Input: part model. Units: mm. Frame: model coordinates. A direction names the side the tool comes from. Give positions to 0.01 mm unless a question says otherwise; leave off trailing zeros. Order: outer loops, then holes, each group sorted by start corner. A loop starts at its lowest first (then second) coordinate and runs counter-clockwise, first axis right, second up. Notation, with made-up numbers: (-4, 64.25) - (20, 64.25) arc R26 ccw to (20, 95.25) - close; hole circle Ø4 at (3.5, 37.25). An arc over 180 degrees is marked (long way). Answer in a Markdown table with one row per item. Add a question column.
from build123d import *

# Parameters (mm, degrees)
CHAMFER_1_SIZE = 1.5


with BuildPart() as part:
    # Эскиз1 → Повернуть1 (revolve)
    with BuildSketch(Plane(origin=(0, 0, 0), x_dir=(0, 0, -1), z_dir=(1, 0, 0))):
        Polygon((-15, 0), (-28.5, 0), (-28.5, 19), (-23.5, 19), (-23.5, 5), (-11, 5), (-11, -5), (-15, -5), align=None)
    revolve(axis=Axis((0, 19.771159875, 0), (0, -1, 0)))

    # Фаска1
    chamfer_1_edges = [part.edges().sort_by_distance(p)[0] for p in [
        (0, 19, -28.5),
        (0, 0, -28.5),
        (0, -5, -15),
    ]]
    chamfer(chamfer_1_edges, length=CHAMFER_1_SIZE)


solid = part.part
Q1. Section C-C, the plane y = 15. Return loops of the section in (x, z).
Q2. Pull-direction query (Z, two-part tool) for faces 3 (the cylindrical face through (-0.66, -1.726, -14.985)), 4 (the flat face through (12, 0, -12)), 5 (the cylindrical face through (10.74, -0.07, -2.38)), 6 (the flat face through (5, 5, 10)); classes: +Z half, -Z half, draft (parallel to the pull), parting line (faces both ways), or undercut.
Q3. Section A-A, the plane x = 0. Return loops of the section in (y, z).
Q4. Access query for faces 1 (the cylindrical face through (-7.1, 11.9, 22.4)), 2 (the cylindrical face through (10.916, 9.612, 26.327)). Directions: +Z, -Z, +X, -X, +Y, -Y. A direction counts if a zero-diameter tool reaches every point of the face in a straight line with its end or side. Return the directions, or none.
Q5. Line query: probe 1 along Z at (x, y) = (0, 12); probe 2 along Z at (x, y) = (0, -1). Output: solid intervals per line, ascending.
Q6. Contact query for flat-ended pins moving along their axis: P1, Ø4, axis at x = 20, z = 14, coming from the -Y side; P2, Ø10, axis at y = 15, z = 18.5, coming from the +X side; P3, Ø6, axis at y = -1, z = -7, coming from the +X side; P4, Ø20, axis at x = 0, z = 0, coming from the +Y side. Output: stop coordinate, or through.
Q7. Section B-B, the plane z = 0. Return loops of the section in (x, y), then the cut area to 3 significant figures.
Computed:
| question | item | result |
|---|---|---|
| 1 | outline | circle Ø57 at (0, 0); hole circle Ø47 at (0, 0) |
| 2 | face 3 | parting line |
| 2 | face 4 | draft |
| 2 | face 5 | undercut |
| 2 | face 6 | undercut |
| 3 | outline | (-5, -13.5) - (-3.5, -15) - (0, -15) - (0, -27) - (1.5, -28.5) - (17.5, -28.5) - (19, -27) - (19, -23.5) - (5, -23.5) - (5, -11) - (-5, -11) - close; (-5, 11) - (5, 11) - (5, 23.5) - (19, 23.5) - (19, 27) - (17.5, 28.5) - (1.5, 28.5) - (0, 27) - (0, 15) - (-3.5, 15) - (-5, 13.5) - close |
| 4 | face 1 | +Y |
| 4 | face 2 | +Y, -Y |
| 5 | probe 1 | z = -28.5 to -23.5, 23.5 to 28.5 |
| 5 | probe 2 | z = -15 to -11, 11 to 15 |
| 6 | P1 | stops at y = 0 |
| 6 | P2 | stops at x = 25.1 |
| 6 | P3 | stops at x = 27.99 |
| 6 | P4 | passes through |
| 7 | outline | (-28.5, 1.5) - (-27, 0) - (-15, 0) - (-15, -3.5) - (-13.5, -5) - (-11, -5) - (-11, 5) - (-23.5, 5) - (-23.5, 19) - (-27, 19) - (-28.5, 17.5) - close; (11, -5) - (13.5, -5) - (15, -3.5) - (15, 0) - (27, 0) - (28.5, 1.5) - (28.5, 17.5) - (27, 19) - (23.5, 19) - (23.5, 5) - (11, 5) - close |
| 7 | area | 348 mm^2 |
